from build123d import *

# Parameters (mm, degrees)
SKETCH1_W           = 100
SKETCH1_H           = 10
BOSS_EXTRUDE1_DEPTH = 1.5
SKETCH2_R           = 1
CUT_EXTRUDE2_DEPTH  = 2
SKETCH5_W           = 1.5
SKETCH5_H           = 2
SKETCH5_W_2         = 4.5
CUT_EXTRUDE4_DEPTH  = 2


with BuildPart() as part:
    # Sketch1 → Boss-Extrude1 (new body)
    with BuildSketch(Plane(origin=(0, 0, 0), x_dir=(1, 0, 0), z_dir=(0, 1, 0))):
        with Locations((40.170187286, 0.880693734)):
            Rectangle(SKETCH1_W, SKETCH1_H)
    extrude(amount=BOSS_EXTRUDE1_DEPTH)

    # Sketch2 → Cut-Extrude2 (cut)
    with BuildSketch(Plane(origin=(0, 1.5, 0), x_dir=(1, 0, 0), z_dir=(0, 1, 0))):
        with Locations(Location((40.170187286, 0.880693734, 0), (0, 0, 270))):
            Circle(SKETCH2_R)
    extrude(amount=-CUT_EXTRUDE2_DEPTH, mode=Mode.SUBTRACT)

    # Sketch5 → Cut-Extrude4 (cut)
    with BuildSketch(Plane(origin=(0, 1.5, 0), x_dir=(1, 0, 0), z_dir=(0, 1, 0))):
        with Locations((-4.079812714, 4.880693734)):
            Rectangle(SKETCH5_W, SKETCH5_H)
        with Locations((40.170187286, 4.880693734)):
            Rectangle(SKETCH5_W_2, SKETCH5_H)
        with Locations((84.420187286, 4.880693734)):
            Rectangle(SKETCH5_W, SKETCH5_H)
        with Locations((-4.079812714, -3.119306266)):
            Rectangle(SKETCH5_W, SKETCH5_H)
        with Locations((40.170187286, -3.119306266)):
            Rectangle(SKETCH5_W_2, SKETCH5_H)
        with Locations((84.420187286, -3.119306266)):
            Rectangle(SKETCH5_W, SKETCH5_H)
    extrude(amount=-CUT_EXTRUDE4_DEPTH, mode=Mode.SUBTRACT)


solid = part.part
Read the model definition and answer for the solid it produces. Units are mm, in the model's axes. Coordinates: 2 decimals unless noted, no trailing zeros. Order: outer loops, then holes, each group sorted by start corner. A loop starts at its lowest first (then second) coordinate and runs counter-clockwise, first axis right, second up. Notation, with made-up numbers: M -24,-8 L 35,-8 A17 ccw 35,2 Z; hole C 46,60.25 d4. An arc over 180 degrees is marked long. Put each result on its own line as item: value. Start each with the question number.
Item 1: Consider probe 1 along X at (y, z) = (1.3, 2.75); probe 2 along X at (y, z) = (0.8, -1); probe 3 along X at (y, z) = (1.4, -1.5). Determine where each line is inside the solid, lowest interval first. Write a range as [from, to].
Item 2: Given pin 1 Ø0.8 at (x, y) = (-4, 1) entering from -Z; pin 2 Ø0.8 at (x, y) = (41, 1) entering from +Z; pin 3 Ø1.5 at (x, z) = (65, -3) entering from -Y, each flat-ended and moving along its own axis, determine where each tip first touches the part or whether it passes through.
Item 3: The mould has two halves that part along X. Classify faces 1 (the face through (41.01, 0.76, -0.34)), 2 (the face through (39, 0, 0)): +X half, -X half, draft (parallel to the pull), parting line (faces both ways), or undercut.
Item 4: Section A-A, the plane z = -4.75 is taken. Determine the outline of the cut face in (x, y), plus the area to 3 significant figures.
Computed:
1. probe 1: x = [-9.83, -4.83], [-3.33, 37.92], [42.42, 83.67], [85.17, 90.17]
1. probe 2: x = [-9.83, 39.18], [41.16, 90.17]
1. probe 3: x = [-9.83, 39.39], [40.96, 90.17]
2. pin 1: stops at z = -3.88
2. pin 2: stops at z = 2.12
2. pin 3: stops at y = 0
3. face 1: undercut
3. face 2: draft
4. outline: M -9.83,0 L -4.83,0 L -4.83,1.5 L -9.83,1.5 Z; M -3.33,0 L 37.92,0 L 37.92,1.5 L -3.33,1.5 Z; M 42.42,0 L 83.67,0 L 83.67,1.5 L 42.42,1.5 Z; M 85.17,0 L 90.17,0 L 90.17,1.5 L 85.17,1.5 Z
4. area: 139 mm2
